Autodesk Inventor part; units mm, degrees
ref_plane "YZ Plane" through (0, 0, 0) normal (1, 0, 0) x (0, 1, 0)
ref_plane "XZ Plane" through (0, 0, 0) normal (0, 1, 0) x (-1, 0, 0)
ref_plane "XY Plane" through (0, 0, 0) normal (0, 0, 1) x (1, 0, 0)
sketch "Sketch1" plane through (0, 0, 0) normal (0, 1, 0) x (-1, 0, 0)
  circle A0 centre (0, 0) radius 2.875
  circle A1 centre (0, 0) radius 6
  dimension "d0" = 5.75
  dimension "d1" = 12
extrude "Extrusion1" add sketch "Sketch1" along normal blind 0.6
sketch "Sketch2" plane through (0, 0.6, 0) normal (0, 1, 0) x (1, 0, 0)
  circle A0 centre (0, 0) radius 2.875
  circle A1 centre (0, 0) radius 6
  circle A2 centre (0, 0) radius 3.375
  dimension "d4" = 0.5
extrude "Extrusion2" add sketch "Sketch2" along normal blind 0.6 contours A2
chamfer "Chamfer1" distance 0.6 angle 45 1 edges at (-3.375, 0.6, 0)
properties part number "m5_shim_alt"
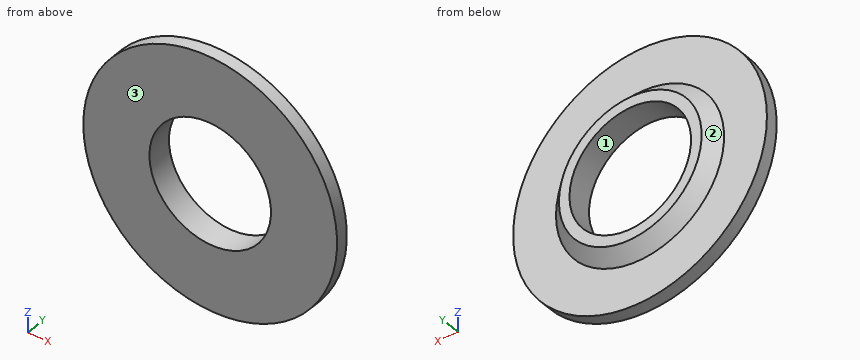
For this review, take the finished solid that the model builds, in its own axes (mm). Face numbers are marked on the shaded views. Round coordinates to 2 decimals unless told otherwise and drop trailing zeros. Write each loop counter-clockwise with the first axis right and the second up, starting at its lowest first coordinate (ties: lowest second). Pieces come first, ordered by that corner, then holes. Notation, with made-up numbers: M 5,27 L 39,27 A20 ccw 39,57 Z; hole C -29,37 d10. An arc over 180 degrees is marked long. Write item = value, one per line. Start each with the question number.
(1) Clearance check with a flat-ended pin moving along its axis: pin 1 Ø5 at (x, z) = (0.5, -4) entering from +Y. State where the tip first meets the part, or that it passes through.
(2) We need section B-B (y = 0.45). Give the boundary of the cut face in (x, z) (3 decimals), then the cut area to 3 significant figures.
(3) The part is to be moulded in two halves that separate along Z. For the marked faces 1, 2 and 3, say which applies: +Z half, -Z half, draft (parallel to the pull), parting line (faces both ways), or undercut.
(4) We need section D-D (z = 4.25). Give the boundary of the cut face in (x, y), then the cut area to 3 significant figures.
(5) For line 1 along Z through (x, y) = (0, 0.55) (3 decimals); line 2 along Z through (x, y) = (-1.75, 1.15); line 3 along X through (y, z) = (0.95, 0) (1 decimal), list the stretches that pass through material, from the lowest coordinate up.
(6) We need section C-C (z = -5). Give the boundary of the cut face in (x, y), then the cut area to 3 significant figures.
Results found:
q1.pin_1 = 1.2
q2.outline = C 0,0 d12; hole C 0,0 d5.75
q2.area = 87.1 mm²
q3.face_1 = undercut
q3.face_2 = parting line
q3.face_3 = draft
q4.outline = M -4.24,0 L 4.24,0 L 4.24,0.6 L -4.24,0.6 Z
q4.area = 5.08 mm²
q5.line_1 = -6 to -2.875, 2.875 to 6
q5.line_2 = -2.94 to -2.28, 2.28 to 2.94
q5.line_3 = -3.6 to -2.9, 2.9 to 3.6
q6.outline = M -3.32,0 L 3.32,0 L 3.32,0.6 L -3.32,0.6 Z
q6.area = 3.98 mm²
